```python
from build123d import *

# Parameters (mm, degrees)
F1_DEPTH = 124.46
F3_DEPTH = 124.46
F4_R     = 1


with BuildPart() as f1:
    # F0 (on Front) → F1 (new body)
    with BuildSketch(Plane.XZ):
        Polygon((-25, 0), (0, 0), (0, 54.543561), align=None)
    extrude(amount=F1_DEPTH)

    # F2 (on face) → F3 (cut, through all)
    with BuildSketch(Plane.XZ.offset(124.46)):
        Polygon((-5.08, 31.189688), (-17.047356, 5.08), (-5.08, 5.08), align=None)
    extrude(amount=-F3_DEPTH, mode=Mode.SUBTRACT)

    # F4
    f4_edges = [f1.edges().sort_by_distance(p)[0] for p in [
        (0, -62.23, 54.543561),
        (-12.5, 0, 27.27178),
        (-25, -62.23, 0),
        (-12.5, -124.46, 27.27178),
        (-12.5, -124.46, 0),
        (0, -124.46, 27.27178),
        (-11.063678, -124.46, 5.08),
        (-11.063678, -124.46, 18.134844),
        (-5.08, -124.46, 18.134844),
        (-12.5, 0, 0),
        (0, -62.23, 0),
        (-5.08, 0, 18.134844),
        (-11.063678, 0, 5.08),
        (-11.063678, 0, 18.134844),
        (0, 0, 27.27178),
    ]]
    fillet(f4_edges, radius=F4_R)


solid = f1.part
```
Read the model definition and answer for the solid it produces. Units are mm, in the model's axes. A direction names the side the tool comes from. Round coordinates to 2 decimals unless told otherwise and drop trailing zeros. Loops run counter-clockwise (first coordinate to the right, second up) from the corner with the lowest first, then second, coordinate; pieces in that order, holes last. Notation, with made-up numbers: (48, 14) -> (99, 14) arc R18 cw to (99, 29) -> close; hole circle Ø3 at (3, 86.25). An arc over 180 degrees is marked (long way). One line per item, written item: value.
1) The mould has two halves that part along Z. Classify faces 1 (the face through (-12.973, -61.373, 26.24)), 2 (the face through (-10.809, -124.175, 19.413)), 3 (the face through (-12, -61, 0)): pulls with the +Z half, pulls with the -Z half, needs draft (parallel to the pull), parting line crosses it, or undercut.
Answer list:
face 1: pulls with the +Z half
face 2: undercut
face 3: pulls with the -Z half
2) For faces 4 (the face through (-13, -124.2, 25.4)), 5 (the face through (-10.8, -0.3, 19.4)), 6 (the face through (-11, -63, 5.08)), determine the directions among +Z, -Z, +X, -X, +Y, -Y from which every point of the face is accessible in a straight line to the end or side of a thin tool.
Answer list:
face 4: +Z, -X, -Y
face 5: +Y
face 6: +Y, -Y
3) A cutting plane is placed at A-A (y = -57.5). Determine the outline of the cut face in (x, z).
Answer list:
outline: (-24.35, 1.42) arc R1 ccw to (-23.44, 0) -> (-1, 0) arc R1 ccw to (0, 1) -> (0, 49.96) arc R1 ccw to (-1.91, 50.38) -> close; hole (-17.05, 5.08) -> (-5.08, 5.08) -> (-5.08, 31.19) -> close
4) Flat-ended cylindrical pins translate along their axes: P1, Ø1, axis at x = -7, y = -17, coming from the +Z side; P2, Ø21, axis at y = -72.5, z = 15, coming from the -X side; P3, Ø8, axis at y = -21, z = 12.5, coming from the -X side; P4, Ø1.5, axis at x = -11, z = 15, coming from the -Y side. Find the tip coordinate at first contact, or state that the pin passes through.
Answer list:
P1: stops at z = 40.36
P2: stops at x = -22.94
P3: stops at x = -21.1
P4: passes through
5) Consider L1, parallel to X at y = -55, z = 43.5; L2, parallel to Z at x = -15, y = -36.5; L3, parallel to X at y = -71, z = 12.5. Determine where each line is inside the solid, lowest interval first. Write a range as [from, to].
Answer list:
L1: x = [-5.06, 0]
L2: z = [0, 5.08], [9.55, 21.82]
L3: x = [-19.27, -13.65], [-5.08, 0]
